Here's how the part is built. I have some questions about the finished solid (model axes, mm). A direction names the side the tool comes from. Give positions to 0.01 mm unless a question says otherwise; leave off trailing zeros. Write each loop counter-clockwise with the first axis right and the second up, starting at its lowest first coordinate (ties: lowest second). Pieces come first, ordered by that corner, then holes. Notation, with made-up numbers: M 11,58 L 39,58 A13 cw 39,78 Z; hole C 40,23.5 d10. An arc over 180 degrees is marked long. Use one line per item in the form item = value. Start each with the question number.
from build123d import *

# Parameters (mm, degrees)
F0_W     = 19.05
F0_H     = 19.05
F1_DEPTH = 1.6383
F2_R     = 1.5875
F3_R     = 1
F4_DEPTH = 1.6393
F5_W     = 4
F5_H     = 4
F6_DEPTH = 1.45


with BuildPart() as f1:
    # F0 (on Top) → F1 (new body)
    with BuildSketch(Plane.XY):
        Rectangle(F0_W, F0_H)
    extrude(amount=F1_DEPTH)

    # F2
    f2_edges = [f1.edges().sort_by_distance(p)[0] for p in [
        (-9.525, 9.525, 0.81915),
        (9.525, 9.525, 0.81915),
        (9.525, -9.525, 0.81915),
        (-9.525, -9.525, 0.81915),
    ]]
    fillet(f2_edges, radius=F2_R)

    # F3 (on face) → F4 (cut, through all)
    with BuildSketch(Plane.XY.offset(1.6383)):
        with Locations((-6.985, 6.985)):
            Circle(F3_R)
        with Locations((-6.985, -6.985)):
            Circle(F3_R)
    extrude(amount=-F4_DEPTH, mode=Mode.SUBTRACT)

    # F5 (on face) → F6 (join)
    with BuildSketch(Plane.XY.offset(1.6383)):
        Rectangle(F5_W, F5_H)
    extrude(amount=F6_DEPTH)


solid = f1.part
1) Thinking about a two-plate mould opening in Y: for faces 1 (the face through (-7.115, 7.976, 0.831)), 2 (the face through (-7.2, -7.96, 0.83)), 3 (the face through (9.07, 9.05, 0.83)), 4 (the face through (0, 0, 3.088)), which applies, released by +Y, released by -Y, zero draft, split by the parting line, or undercut?
2) Will these pins go through, and if not, where does the flat tip stop? P1, Ø1.2, axis at y = 0.5, z = 2, coming from the +X side (3 decimals); P2, Ø5, axis at x = -5, y = 7.5, coming from the +Z side; P3, Ø1.6, axis at x = 0.5, z = 2.5, coming from the -Y side; P4, Ø1.2, axis at y = 0, z = 2.5, coming from the -X side.
3) Suppose I cut it at B-B, the plane y = 6.25. List the corners of the cut face in (x, z) for me (3 decimals).
4) Suppose I cut it at C-C, the plane z = 1.25. List the corners of the cut face in (x, y) for me (1 decimal).
5) Please list where these lines run through material, in increasing order: line 1 (Y direction, x = -7.75, z = 1.45) (3 decimals); line 2 (Z direction, x = -2.5, y = 2.5); line 3 (Y direction, x = -1, z = 2.55).
6) On a 3-axis mill with a long thin cutter (end or side, diameter ignored), from which of +Z, -Z, +X, -X, +Y, -Y can I reach the whole of each face in a straight line? I mean faces 5 (the face through (2, 0, 2)), 6 (the face through (0, 2, 2)), 7 (the face through (-2, 0, 2)), 8 (the face through (0, -2, 2)). Say none if no direction works.
7) Suppose I cut it at A-A, the plane x = 1.5. List the corners of the cut face in (y, z) for me (3 decimals).
Checks:
q1.face_1 = undercut
q1.face_2 = undercut
q1.face_3 = released by +Y
q1.face_4 = zero draft
q2.P1 = 9.525
q2.P2 = 1.64
q2.P3 = -2
q2.P4 = -2
q3.outline = M -9.525,0 L -7.663,0 L -7.663,1.638 L -9.525,1.638 Z; M -6.307,0 L 9.525,0 L 9.525,1.638 L -6.307,1.638 Z
q4.outline = M -9.5,-7.9 A1.6 ccw -7.9,-9.5 L 7.9,-9.5 A1.6 ccw 9.5,-7.9 L 9.5,7.9 A1.6 ccw 7.9,9.5 L -7.9,9.5 A1.6 ccw -9.5,7.9 Z; hole C -7,-7 d2; hole C -7,7 d2
q5.line_1 = -9.525 to -7.629, -6.341 to 6.341, 7.629 to 9.525
q5.line_2 = 0 to 1.64
q5.line_3 = -2 to 2
q6.face_5 = +Z, +X, +Y, -Y
q6.face_6 = +Z, +X, -X, +Y
q6.face_7 = +Z, -X, +Y, -Y
q6.face_8 = +Z, +X, -X, -Y
q7.outline = M -9.525,0 L 9.525,0 L 9.525,1.638 L 2,1.638 L 2,3.088 L -2,3.088 L -2,1.638 L -9.525,1.638 Z
